```python
from build123d import *

# Parameters (mm, degrees)
SKETCH1_W           = 42.7
SKETCH1_H           = 22.7
SKETCH1_R           = 4
SKETCH1_R_2         = 1
BOSS_EXTRUDE1_DEPTH = 1
SKETCH2_W           = 1
SKETCH2_H           = 22.7
BOSS_EXTRUDE2_DEPTH = 26
SKETCH3_W           = 39.7
SKETCH3_H           = 1
BOSS_EXTRUDE3_DEPTH = 4.6
FILLET2_R           = 1
SKETCH4_R           = 4
SKETCH4_R_2         = 1
CUT_EXTRUDE1_DEPTH  = 1
CUT_EXTRUDE2_START  = -1
SKETCH5_R           = 1
SKETCH5_R_2         = 4
CUT_EXTRUDE2_DEPTH  = 1


with BuildPart() as part:
    # Sketch1 → Boss-Extrude1 (new body)
    with BuildSketch(Plane(origin=(0, 0, 0), x_dir=(1, 0, 0), z_dir=(0, 1, 0))):
        with Locations((21.35, 11.35)):
            Rectangle(SKETCH1_W, SKETCH1_H)
        with Locations(Location((21.35, 11.35, 0), (0, 0, 270))):
            Circle(SKETCH1_R, mode=Mode.SUBTRACT)
        with Locations(Location((26.299747468, 16.299747468, 0), (0, 0, 270))):
            Circle(SKETCH1_R_2, mode=Mode.SUBTRACT)
        with Locations(Location((26.299747468, 6.400252532, 0), (0, 0, 270))):
            Circle(SKETCH1_R_2, mode=Mode.SUBTRACT)
        with Locations(Location((16.400252532, 6.400252532, 0), (0, 0, 270))):
            Circle(SKETCH1_R_2, mode=Mode.SUBTRACT)
        with Locations(Location((16.400252532, 16.299747468, 0), (0, 0, 270))):
            Circle(SKETCH1_R_2, mode=Mode.SUBTRACT)
    extrude(amount=BOSS_EXTRUDE1_DEPTH)

    # Sketch2 → Boss-Extrude2 (add)
    with BuildSketch(Plane(origin=(0, 1, 0), x_dir=(1, 0, 0), z_dir=(0, 1, 0))):
        with Locations((0.5, 11.35)):
            Rectangle(SKETCH2_W, SKETCH2_H)
        with Locations((42.2, 11.35)):
            Rectangle(SKETCH2_W, SKETCH2_H)
    extrude(amount=BOSS_EXTRUDE2_DEPTH)

    # Sketch3 → Boss-Extrude3 (add)
    with BuildSketch(Plane(origin=(0, 1, 0), x_dir=(1, 0, 0), z_dir=(0, 1, 0))):
        with Locations((21.35, 22.2)):
            Rectangle(SKETCH3_W, SKETCH3_H)
        with Locations((21.35, 0.5)):
            Rectangle(SKETCH3_W, SKETCH3_H)
    extrude(amount=BOSS_EXTRUDE3_DEPTH)

    # Fillet2
    fillet2_edges = [part.edges().sort_by_distance(p)[0] for p in [
        (42.7, 0, -11.35),
        (0, 0, -11.35),
    ]]
    fillet(fillet2_edges, radius=FILLET2_R)

    # Sketch4 → Cut-Extrude1 (cut)
    with BuildSketch(Plane.ZY):
        with Locations((-11.35, 16.5)):
            Circle(SKETCH4_R)
        with Locations((-18.774621202, 23.924621202)):
            Circle(SKETCH4_R_2)
        with Locations((-3.925378798, 23.924621202)):
            Circle(SKETCH4_R_2)
        with Locations((-3.925378798, 9.075378798)):
            Circle(SKETCH4_R_2)
        with Locations((-18.774621202, 9.075378798)):
            Circle(SKETCH4_R_2)
    extrude(amount=-CUT_EXTRUDE1_DEPTH, mode=Mode.SUBTRACT)

    # Sketch5 → Cut-Extrude2 (cut)
    with BuildSketch(Plane(origin=(42.7, 0, 0), x_dir=(0, 0, -1), z_dir=(1, 0, 0)).offset(CUT_EXTRUDE2_START)):
        with BuildLine():
            Line((0, 27), (0, 15.65))
            ThreePointArc((0, 15.65), (3.324338034, 23.675661966), (11.35, 27))
            Line((11.35, 27), (0, 27))
        make_face()
        with BuildLine():
            Line((22.7, 27), (11.35, 27))
            ThreePointArc((11.35, 27), (19.375661966, 23.675661966), (22.7, 15.65))
            Line((22.7, 15.65), (22.7, 27))
        make_face()
        with Locations((11.35, 23.3)):
            Circle(SKETCH5_R)
        with Locations(Location((11.35, 16.5, 0), (0, 0, 180))):
            Circle(SKETCH5_R_2)
        with Locations((18.15, 16.5)):
            Circle(SKETCH5_R)
        with Locations((11.35, 9.7)):
            Circle(SKETCH5_R)
        with Locations((4.55, 16.5)):
            Circle(SKETCH5_R)
    extrude(amount=CUT_EXTRUDE2_DEPTH, mode=Mode.SUBTRACT)


solid = part.part
```
Geometry check sheet. Reference: the model listing, model coordinates, mm. A direction names the side the tool comes from. Give positions to 0.01 mm unless a question says otherwise; leave off trailing zeros. Loops run counter-clockwise (first coordinate to the right, second up) from the corner with the lowest first, then second, coordinate; pieces in that order, holes last. Notation, with made-up numbers: (77.5, 10) - (108.5, 10) arc R9 cw to (108.5, 20) - close; hole circle Ø9 at (18, 59). An arc over 180 degrees is marked (long way). Use CSV: the item, a comma, the result in double quotes. Start each with the question number.
Q1. Section check D-D, the plane z = -9.75. Record the cut outline in (x, y).
Q2. Release check for a two-part mould opening along X. For faces 1 (the face through (26, 0, -12)), 2 (the face through (0, 11, -11)), 3 (the face through (21.1, 5.6, -0.5)) record: +X half, -X half, draft (parallel to the pull), parting line (faces both ways), or undercut.
Q3. Go/stop test with a flat-tipped pin: pin 1 Ø1.2 at (y, z) = (16.5, -18.15) entering from +X. Record where the tip stops, or that it passes through.
Q4. Access from +Z, -Z, +X, -X, +Y, -Y to the whole of each face (thin tool, end or side, straight path). Record for faces 4 (the face through (42.19, 10.54, -11.89)), 5 (the face through (16.4, 0.5, -17.3)), 6 (the face through (21, 3, -21.7)), 7 (the face through (41.2, 3.3, -0.5)), 8 (the face through (0.49, 23.32, -19.57)).
Q5. Section check C-C, the plane y = 2.25. Record the cut outline in (x, z).
Q6. Section check B-B, the plane x = 21.35. Record the cut outline in (y, z).
Q7. Section check A-A, the plane y = 11.5. Record the cut outline in (x, z), and give its area (3 significant figures).
Q8. Scan lines: probe 1 along X at (y, z) = (24.25, -13.75); probe 2 along Y at (x, z) = (42.3, -11.35); probe 3 along Z at (x, y) = (23.5, 2.25). Record each from-to range of solid material in increasing order. Write a range as from..to.
Findings below:
1,outline,"(0, 1) arc R1 ccw to (1, 0) - (17.68, 0) - (17.68, 1) - (1, 1) - (1, 12.83) - (0, 12.83) - close; (0, 20.17) - (1, 20.17) - (1, 27) - (0, 27) - close; (25.02, 0) - (41.7, 0) arc R1 ccw to (42.7, 1) - (42.7, 12.83) - (41.7, 12.83) - (41.7, 1) - (25.02, 1) - close; (41.7, 20.17) - (42.7, 20.17) - (42.7, 26.89) - (41.7, 26.89) - close"
2,face 1,"draft"
2,face 2,"-X half"
2,face 3,"undercut"
3,pin 1,"stops at x = 1"
4,face 4,"+X"
4,face 5,"+Y, -Y"
4,face 6,"+Y"
4,face 7,"+Z, -Z, +Y"
4,face 8,"-X"
5,outline,"(0, -22.7) - (1, -22.7) - (1, 0) - (0, 0) - close; (1.5, -22.7) - (41.2, -22.7) - (41.2, -21.7) - (1.5, -21.7) - close; (1.5, -1) - (41.2, -1) - (41.2, 0) - (1.5, 0) - close; (41.7, -22.7) - (42.7, -22.7) - (42.7, 0) - (41.7, 0) - close"
6,outline,"(0, -22.7) - (5.6, -22.7) - (5.6, -21.7) - (1, -21.7) - (1, -15.35) - (0, -15.35) - close; (0, -7.35) - (1, -7.35) - (1, -1) - (5.6, -1) - (5.6, 0) - (0, 0) - close"
7,outline,"(0, -22.7) - (1, -22.7) - (1, 0) - (0, 0) - close; (41.7, -22.7) - (42.7, -22.7) - (42.7, 0) - (41.7, 0) - close"
7,area,"45.4 mm^2"
8,probe 1,"x = 0..1, 41.7..42.7"
8,probe 2,"y = 0.2..8.7, 10.7..12.5, 20.5..22.3, 24.3..27"
8,probe 3,"z = -22.7..-21.7, -1..0"
